```python
from build123d import *


with BuildPart() as f2:
    # F2: sweep along a path in F1
    with BuildLine(Plane.XZ) as f2_path:
        Line((0, 0), (287.6, 0))
        Line((287.6, 0), (487.6, 200))
        Line((487.6, 200), (487.6, 1000))
        Line((487.6, 1000), (-487.6, 1000))
        Line((-487.6, 1000), (-487.6, 0))
        Line((-487.6, 0), (0, 0))
    # F0 (on Right) → F2 (sweep)
    with BuildSketch(Plane.YZ):
        Polygon((-163.6, 76.4), (-201.6, 76.4), (-201.6, 0), (0, 0), (0, 104.8), (-163.6, 104.8), align=None)
    sweep(path=f2_path.line, transition=Transition.RIGHT)


solid = f2.part
```
Read the model definition and answer for the solid it produces. Units are mm, in the model's axes. A direction names the side the tool comes from. Coordinates: 2 decimals unless noted, no trailing zeros. Write each loop counter-clockwise with the first axis right and the second up, starting at its lowest first coordinate (ties: lowest second). Pieces come first, ordered by that corner, then holes. Notation, with made-up numbers: (-22.75, -11.5) -> (14.25, -11.5) arc R26 ccw to (14.25, 26.5) -> close; hole circle Ø1 at (59.5, 28). An arc over 180 degrees is marked (long way). Write item = value, one per line.
(1) Section C-C on x = 100 is taken. Write down the section's boundary in (y, z).
From the geometry:
outline = (-201.6, 0) -> (0, 0) -> (0, 104.8) -> (-163.6, 104.8) -> (-163.6, 76.4) -> (-201.6, 76.4) -> close; (-201.6, 923.6) -> (-163.6, 923.6) -> (-163.6, 895.2) -> (0, 895.2) -> (0, 1000) -> (-201.6, 1000) -> close
(2) For a pull along X with two mould halves and no side action, classify faces 4 (the face through (-411.2, -182, 494)), 5 (the face through (-487.6, -102, 493)), 6 (the face through (-95, -102, 0)), 7 (the face through (-382.8, -81, 494)) as +X half, -X half, draft (parallel to the pull), parting line (faces both ways), or undercut.
From the geometry:
face_4 = undercut
face_5 = -X half
face_6 = draft
face_7 = undercut
(3) Given pin 1 Ø19 at (x, y) = (199.5, -189.5) entering from -Z, flat-ended and moving along its own axis, determine where the tip first touches the part or whether it passes through.
From the geometry:
pin_1 = 0
(4) Straight lines are drawn through the part: L1, parallel to Z at x = 185.5, y = -187; L2, parallel to Z at x = 153.5, y = -54.5; L3, parallel to X at y = -177, z = 714. For each, find the intervals that lie inside material, in ascending order. Write a range as from..to.
From the geometry:
L1 = 0..76.4, 923.6..1000
L2 = 0..104.8, 895.2..1000
L3 = -487.6..-411.2, 411.2..487.6
(5) Which of the six approach directions +Z, -Z, +X, -X, +Y, -Y give full straight-line access (tool end or side, diameter ignored) to faces 1 (the face through (-73, -182, 76.4)), 2 (the face through (314.47, -80.65, 175.08)), 3 (the face through (487.6, -102, 606))?
From the geometry:
face_1 = -Y
face_2 = +Y, -Y
face_3 = +Z, -Z, +X, +Y, -Y
(6) Section B-B on y = -19.5 is taken. Write down the section's boundary in (x, z).
From the geometry:
outline = (-487.6, 0) -> (287.6, 0) -> (487.6, 200) -> (487.6, 1000) -> (-487.6, 1000) -> close; hole (-382.8, 104.8) -> (244.19, 104.8) -> (382.8, 243.41) -> (382.8, 895.2) -> (-382.8, 895.2) -> close
(7) Section A-A on z = 327.5 is taken. Write down the section's boundary in (x, y), plus the area to 3 significant figures.
From the geometry:
outline = (-487.6, -201.6) -> (-411.2, -201.6) -> (-411.2, -163.6) -> (-382.8, -163.6) -> (-382.8, 0) -> (-487.6, 0) -> close; (382.8, -163.6) -> (411.2, -163.6) -> (411.2, -201.6) -> (487.6, -201.6) -> (487.6, 0) -> (382.8, 0) -> close
area = 40,100 mm2
